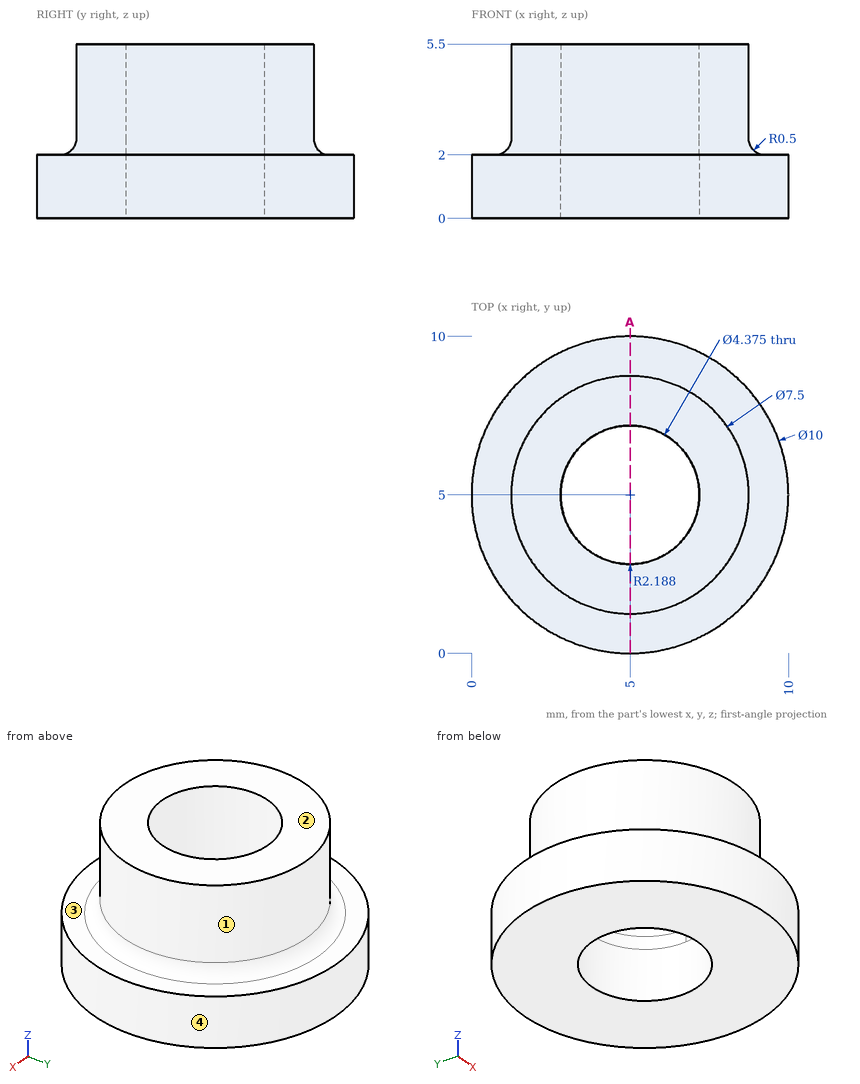
Design review of the part shown in the three views and the two pictorial views. Dimensions are in mm from the part's minimum x, y and z. A direction names the side the tool comes from. Coordinates: 2 decimals unless noted, no trailing zeros. Order: outer loops, then holes, each group sorted by start corner. A loop starts at its lowest first (then second) coordinate and runs counter-clockwise, first axis right, second up.
Item 1: For the marked faces 1 and 2, list the 3-axis set-ups (+Z, -Z, +X, -X, +Y, -Y) from which the entire face can be reached by the end or side of a thin tool; tool diameter is ignored.
Item 2: For pin 1 Ø1 at (x, y) = (7, 5.5) entering from -Z, flat-tipped, find the tip position at first contact; note if it passes through.
Item 3: The part is to be moulded in two halves that separate along X. For the marked faces 3 and 4, say which applies: pulls with the +X half, pulls with the -X half, needs draft (parallel to the pull), parting line crosses it, or undercut.
Item 4: Take a section at A-A, the plane x = 5. Write out the cut boundary in (y, z), then the cut area to 3 significant figures.
Item 5: For line 1 (Y direction, x = 5, z = 1.3); line 2 (Y direction, x = 5, z = 4.4); line 3 (X direction, y = 6.5, z = 5.2) (1 decimal), list the stretches that pass through material, from the lowest coordinate up.
The answers:
1. face 1: +Z
1. face 2: +Z, +X, -X, +Y, -Y
2. pin 1: stops at z = 0
3. face 3: needs draft
3. face 4: parting line crosses it
4. outline: (0, 0) - (2.81, 0) - (2.81, 5.5) - (1.25, 5.5) - (1.25, 2.5) arc R0.5 cw to (0.75, 2) - (0, 2) - close; (7.19, 0) - (10, 0) - (10, 2) - (9.25, 2) arc R0.5 cw to (8.75, 2.5) - (8.75, 5.5) - (7.19, 5.5) - close
4. area: 22.3 mm2
5. line 1: y = 0 to 2.81, 7.19 to 10
5. line 2: y = 1.25 to 2.81, 7.19 to 8.75
5. line 3: x = 1.6 to 3.4, 6.6 to 8.4
